```python
from build123d import *

# Parameters (mm, degrees)
BOSS_EXTRUDE1_DEPTH      = 3.95
SHELL1_START             = -2.75
SHELL1_DEPTH             = 5.5
BOSS_EXTRUDE2_REACH      = 11.943
BOSS_EXTRUDE2_END_RADIUS = 32.700000868
BOSS_EXTRUDE2_START      = 0.02
SKETCH2_R                = 2.3
SKETCH2_R_2              = 1.9
SKETCH3_W                = 6.823927471
SKETCH3_H                = 5.581929969
CUT_EXTRUDE1_DEPTH       = 2.4
BOSS_EXTRUDE3_REACH      = 11.601
BOSS_EXTRUDE3_START      = -0.2
SKETCH4_R                = 2.6
SKETCH4_R_2              = 2.3
CUT_EXTRUDE6_DEPTH       = 10.923471076
CUT_EXTRUDE6_DEPTH_BACK  = 10.923471076


with BuildPart() as part:
    # Sketch1 → Boss-Extrude1 (new, symmetric)
    with BuildSketch(Plane.XY):
        with BuildLine():
            Line((-7.9, 1.037208095), (0, 1.037208095))
            Line((0, 1.037208095), (0, 2.340892579))
            Line((0, 2.340892579), (7.9, 2.340892579))
            Line((7.9, 2.340892579), (7.9, 5.540892579))
            ThreePointArc((7.9, 5.540892579), (-0.199501968, 4.843176285), (-7.9, 2.237208095))
            Line((-7.9, 2.237208095), (-7.9, 1.037208095))
        make_face()
    extrude(amount=BOSS_EXTRUDE1_DEPTH, both=True)

    # Shell1: read off the stored shape, not the designer's step
    # Shell1 outline → Shell1 (cut)
    with BuildSketch(Plane.XY.offset(SHELL1_START)):
        with BuildLine():
            Line((-1.2, 1.037208095), (-1.2, 3.382492095))
            ThreePointArc((-1.2, 3.382492095), (-3.992613389, 2.549753458), (-6.7, 1.471699231))
            Line((-6.7, 1.471699231), (-6.7, 1.037208095))
            Line((-6.7, 1.037208095), (-1.2, 1.037208095))
        make_face()
        with BuildLine():
            ThreePointArc((6.7, 4.360765395), (3.058165542, 4.152993699), (-0.537868318, 3.540892579))
            Line((-0.537868318, 3.540892579), (6.7, 3.540892579))
            Line((6.7, 3.540892579), (6.7, 4.360765395))
        make_face()
    extrude(amount=SHELL1_DEPTH, mode=Mode.SUBTRACT)

    # Boss-Extrude2: up to this cylinder (the profile starts inside it)
    boss_extrude2_end = Plane(origin=(6.738734935, -28.339212532, 2.234946), z_dir=(0, 0, -1)) * Cylinder(BOSS_EXTRUDE2_END_RADIUS, 90.286001737, mode=Mode.PRIVATE)
    # Sketch2 → Boss-Extrude2 (add, up to the surface)
    with BuildSketch(Plane(origin=(0, 1.037208095, 0), x_dir=(-1, 0, 0), z_dir=(0, -1, 0)).offset(BOSS_EXTRUDE2_START), mode=Mode.PRIVATE) as boss_extrude2_sk1:
        with Locations(Location((3.95, 0, 0), (0, 0, 90))):
            Circle(SKETCH2_R)
        with Locations(Location((3.95, 0, 0), (0, 0, 90))):
            Circle(SKETCH2_R_2, mode=Mode.SUBTRACT)
    boss_extrude2_tool1 = extrude(boss_extrude2_sk1.sketch, amount=-BOSS_EXTRUDE2_REACH, mode=Mode.PRIVATE) & boss_extrude2_end
    add(boss_extrude2_tool1.solids().sort_by_distance((-3.95, 1.017208, 2.234946))[0])

    # Sketch3 → Cut-Extrude1 (cut)
    with BuildSketch(Plane.XZ.offset(-2.340892579)):
        with Locations((3.411963736, 0.021143674)):
            Rectangle(SKETCH3_W, SKETCH3_H)
    extrude(amount=-CUT_EXTRUDE1_DEPTH, mode=Mode.SUBTRACT)

    # Sketch4 → Boss-Extrude3 (add, up to next)
    with BuildSketch(Plane(origin=(0, 2.340892579, 0), x_dir=(-1, 0, 0), z_dir=(0, -1, 0)).offset(BOSS_EXTRUDE3_START), mode=Mode.PRIVATE) as boss_extrude3_sk1:
        with Locations(Location((-3.411963735, 0, 0), (0, 0, 90))):
            Circle(SKETCH4_R)
        with Locations(Location((-3.411963735, 0, 0), (0, 0, 90))):
            Circle(SKETCH4_R_2, mode=Mode.SUBTRACT)
    boss_extrude3_tool1 = extrude(boss_extrude3_sk1.sketch, amount=-BOSS_EXTRUDE3_REACH, mode=Mode.PRIVATE) - part.part
    add(boss_extrude3_tool1.solids().sort_by_distance((3.411964, 2.540893, 2.526461))[0])

    # Sketch10 → Cut-Extrude6 (cut, two sides: drawn at the far end of the back side and taken through both)
    with BuildSketch(Plane(origin=(0, 1.037208095, 0), x_dir=(-1, 0, 0), z_dir=(0, -1, 0)).offset(-CUT_EXTRUDE6_DEPTH_BACK)):
        Polygon((7.9, 2.798684465), (0, -3.95), (7.9, -3.95), align=None)
    extrude(amount=CUT_EXTRUDE6_DEPTH + CUT_EXTRUDE6_DEPTH_BACK, mode=Mode.SUBTRACT)


solid = part.part
```
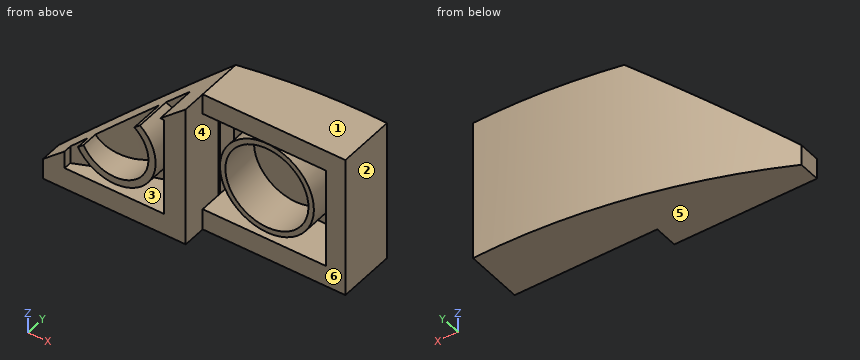
Design review of the part built by this model. Coordinates are the model's own, in mm. Face numbers are marked on the shaded views. A direction names the side the tool comes from. Coordinates: 2 decimals unless noted, no trailing zeros. Write each loop counter-clockwise with the first axis right and the second up, starting at its lowest first coordinate (ties: lowest second). Pieces come first, ordered by that corner, then holes.
1) Add section C-C (z = -3.5). Write out the cut boundary in (x, y), plus the area to 3 significant figures.
2) Machinability: for the marked faces 4, 5 and 6, which of the approach directions +Z, -Z, +X, -X, +Y, -Y give a long, thin tool a straight path to every point of the face, cutting with its end or side? Answer none if there is none.
3) Insertion check: pin 1 (2.5 mm diameter, centred on x = 3, z = 0.5, fed in from -Y); pin 2 (3 mm diameter, centred on x = -1, z = 1, fed in from -Y); pin 3 (1.9 mm diameter, centred on y = 3, z = 0, fed in from -X); pin 4 (2.5 mm diameter, centred on x = -3.95, z = 0, fed in from -Y). Each pin has a flat end and moves straight along its axis. Give the tip position at first contact, or say it passes through.
4) Add section B-B (x = 4.25). Write out the cut boundary in (y, z).
5) To check wall thickness, follow L1, parallel to Z at x = 0.25, y = 3.6; L2, parallel to Z at x = -3.95, y = 1.85; L3, parallel to X at y = 3.2, z = 0. State the ranges of each line that lie inside material, in increasing order.
6) Add section A-A (y = 4). Write out the cut boundary in (x, z).
7) Mouldability with a two-part tool opening along X and no side actions: class the marked faces 1, 2 and 3 as +X half, -X half, draft (parallel to the pull), parting line (faces both ways), or undercut.
8) Add section D-D (x = -3.5). Write out the cut boundary in (y, z), plus the area to 3 significant figures.
Check result:
1. outline: (-7.9, 1.04) - (0, 1.04) - (0, 2.34) - (7.9, 2.34) - (7.9, 5.54) arc R33.9 ccw to (-7.9, 2.24) - close
1. area: 45.3 mm2
2. face 4: -Y
2. face 5: -Z, +X, -X, +Y, -Y
2. face 6: +Z, -Z, +X, -Y
3. pin 1: stops at y = 4.74
3. pin 2: stops at y = 1.02
3. pin 3: stops at x = -5.74
3. pin 4: stops at y = 2.13
4. outline: (2.34, -3.95) - (5.47, -3.95) - (5.47, 3.95) - (2.34, 3.95) - (2.34, 2.81) - (4.74, 2.81) - (4.74, 2.46) - (2.54, 2.46) - (2.54, 2.14) - (4.74, 2.14) - (4.74, -2.14) - (2.54, -2.14) - (2.54, -2.46) - (4.74, -2.46) - (4.74, -2.77) - (2.34, -2.77) - close
5. L1: z = -3.95 to -2.77, 2.81 to 3.95
5. L2: z = -3.95 to -2.75, -2.3 to -1.9
5. L3: x = -4.62 to -1.65, -1.2 to 0, 0.81 to 1.11, 5.71 to 6.01, 6.82 to 7.9
6. outline: (-3.43, -3.95) - (7.9, -3.95) - (7.9, 3.95) - (0, 3.95) - (-3.43, 1.02) - close; circle Ø5.2 at (3.41, 0); hole (0, -2.77) - (6.82, -2.77) - (6.82, 2.81) - (0, 2.81) - close; hole circle Ø4.6 at (3.41, 0)
7. face 1: draft
7. face 2: +X half
7. face 3: undercut
8. outline: (1.02, -2.26) - (2.72, -2.26) - (2.72, -2.75) - (1.04, -2.75) - (1.04, -3.95) - (3.98, -3.95) - (3.98, 0.96) - (2.72, 0.96) - (2.72, -1.85) - (1.02, -1.85) - close
8. area: 8.90 mm2
